from build123d import *

# Parameters (mm, degrees)
SM_BASE_FLANGE_1_DEPTH      = 10
SM_EDGE_FLANGE_2_DEPTH      = 18
SM_START                    = 1
SM_EDGE_FLANGE_2_FLAT_DEPTH = 1


# Sheet-metal steps are written as plain solids
with BuildPart() as part:
    # Sketch 1 → 基体-法兰1 (new body)
    with BuildSketch(Plane.XY):
        with BuildLine():
            Line((0, 0), (18, 0))
            ThreePointArc((18, 0), (19.414213562, 0.585786438), (20, 2))
            Line((20, 2), (20, 15))
            Line((20, 15), (21, 15))
            Line((21, 15), (21, 2))
            ThreePointArc((21, 2), (20.121320344, -0.121320344), (18, -1))
            Line((18, -1), (0, -1))
            Line((0, -1), (0, 0))
        make_face()
    extrude(amount=SM_BASE_FLANGE_1_DEPTH)

    # 边线-法兰2 bend section (across the edge) → 边线-法兰2 (add)
    with BuildSketch(Plane(origin=(18, -1, 32), x_dir=(0, 0, -1), z_dir=(-1, 0, 0))):
        with BuildLine():
            Line((-1, 2), (0, 2))
            ThreePointArc((0, 2), (0.585786438, 0.585786438), (2, 0))
            Line((2, 0), (22, 0))
            Line((22, 0), (22, -1))
            Line((22, -1), (2, -1))
            ThreePointArc((2, -1), (-0.121320344, -0.121320344), (-1, 2))
        make_face()
    extrude(amount=SM_EDGE_FLANGE_2_DEPTH)

    # 边线-法兰2 profile (on flange) → 边线-法兰2 flat (add)
    with BuildSketch(Plane(origin=(0, -1, 32), x_dir=(-1, 0, 0), z_dir=(0, 0, 1)).offset(SM_START)):
        Polygon((0, 2), (0, 10), (-1.8, 12.5), (-16.2, 12.5), (-18, 10), (-18, 2), align=None)
    extrude(amount=-SM_EDGE_FLANGE_2_FLAT_DEPTH)


solid = part.part
Source: CAD feature listing. Evaluate the final solid. Frame: model axes, mm. A direction names the side the tool comes from. Give positions to 0.01 mm unless a question says otherwise; leave off trailing zeros. Write each loop counter-clockwise with the first axis right and the second up, starting at its lowest first coordinate (ties: lowest second). Pieces come first, ordered by that corner, then holes. Notation, with made-up numbers: (65.5, -19.75) -> (102.5, -19.75) arc R34 cw to (102.5, 13.25) -> close; hole circle Ø10 at (89, 19.25). An arc over 180 degrees is marked (long way). Return JSON: item names as keys, results as strings. Group by question number.
1. Section D-D, the plane z = 24. Output: boundary loops of the cut face in (x, y).
2. Section A-A, the plane x = 3.5. Output: boundary loops of the cut face in (y, z).
3. Pin query (flat end, axial travel): pin 1 Ø11.5 at (x, y) = (7.5, -9.5) entering from -Z; pin 2 Ø3.5 at (x, y) = (20, 7) entering from +Z; pin 3 Ø9 at (x, z) = (8.5, 12) entering from -Y. Return the tip coordinate at first contact, or that it passes through.
4. Access query for faces 1 (the face through (9, -8, 33)), 2 (the face through (20, 8, 5)), 3 (the face through (9.13, -0.86, 32.1)), 4 (the face through (9, -8, 32)), 5 (the face through (18, -0.6, 25)). Directions: +Z, -Z, +X, -X, +Y, -Y. A direction counts if a zero-diameter tool reaches every point of the face in a straight line with its end or side. Return the directions, or none.
5. Material intervals for line 1 (Z direction, x = 6.5, y = -6.25); line 2 (X direction, y = 12, z = 2); line 3 (Y direction, x = 5, z = 27), sorted ascending. Write a range as from..to.
6. Section C-C, the plane y = 7. Output: boundary loops of the cut face in (x, z), then the cut area to 3 significant figures.
7. Section B-B, the plane z = 9. Output: boundary loops of the cut face in (x, y).
Determined:
{
 "1": {"outline": "(0, -1) -> (18, -1) -> (18, 0) -> (0, 0) -> close"},
 "2": {"outline": "(-13.5, 32) -> (-3, 32) arc R2 cw to (-1, 30) -> (-1, 0) -> (0, 0) -> (0, 30) arc R3 ccw to (-3, 33) -> (-13.5, 33) -> close"},
 "3": {"pin 1": "stops at z = 32", "pin 2": "stops at z = 10", "pin 3": "stops at y = -1"},
 "4": {"face 1": "+Z, +X, -X, +Y, -Y", "face 2": "+Z, -Z, -X, +Y", "face 3": "+Z, +X, -X, +Y", "face 4": "-Z, +X, -X, -Y", "face 5": "+Z, +X, +Y, -Y"},
 "5": {"line 1": "z = 32..33", "line 2": "x = 20..21", "line 3": "y = -1..0"},
 "6": {"outline": "(20, 0) -> (21, 0) -> (21, 10) -> (20, 10) -> close", "area": "10.0 mm2"},
 "7": {"outline": "(0, -1) -> (18, -1) arc R3 ccw to (21, 2) -> (21, 15) -> (20, 15) -> (20, 2) arc R2 cw to (18, 0) -> (0, 0) -> close"}
}
